```python
from build123d import *

# Parameters (mm, degrees)
SKETCH1_R           = 75
SKETCH1_R_2         = 4.5
BOSS_EXTRUDE1_DEPTH = 10
SKETCH2_R           = 30
BOSS_EXTRUDE2_DEPTH = 55
SKETCH3_R           = 40
BOSS_EXTRUDE3_DEPTH = 5
SKETCH4_R           = 22.5
CUT_EXTRUDE1_DEPTH  = 60
FILLET1_R           = 5
SKETCH5_W           = 40
SKETCH5_H           = 75
BOSS_EXTRUDE4_DEPTH = 45
CUT_EXTRUDE2_DEPTH  = 113.5
SKETCH7_R           = 30
BOSS_EXTRUDE5_DEPTH = 15
FILLET2_R           = 5
CUT_EXTRUDE3_DEPTH  = 45


with BuildPart() as part:
    # Sketch1 → Boss-Extrude1 (new body)
    with BuildSketch(Plane(origin=(0, 0, 0), x_dir=(1, 0, 0), z_dir=(0, 1, 0))):
        Circle(SKETCH1_R)
        with Locations((37.5, 37.5)):
            Circle(SKETCH1_R_2, mode=Mode.SUBTRACT)
        with Locations((-37.5, 37.5)):
            Circle(SKETCH1_R_2, mode=Mode.SUBTRACT)
        with Locations((-37.5, -37.5)):
            Circle(SKETCH1_R_2, mode=Mode.SUBTRACT)
        with Locations((37.5, -37.5)):
            Circle(SKETCH1_R_2, mode=Mode.SUBTRACT)
    extrude(amount=BOSS_EXTRUDE1_DEPTH)

    # Sketch2 → Boss-Extrude2 (add)
    with BuildSketch(Plane(origin=(0, 10, 0), x_dir=(1, 0, 0), z_dir=(0, 1, 0))):
        Circle(SKETCH2_R)
    extrude(amount=BOSS_EXTRUDE2_DEPTH)

    # Sketch3 → Boss-Extrude3 (add)
    with BuildSketch(Plane(origin=(0, 65, 0), x_dir=(1, 0, 0), z_dir=(0, 1, 0))):
        Circle(SKETCH3_R)
    extrude(amount=BOSS_EXTRUDE3_DEPTH)

    # Sketch4 → Cut-Extrude1 (cut)
    with BuildSketch(Plane(origin=(0, 70, 0), x_dir=(1, 0, 0), z_dir=(0, 1, 0))):
        Circle(SKETCH4_R)
    extrude(amount=-CUT_EXTRUDE1_DEPTH, mode=Mode.SUBTRACT)

    # Fillet1
    fillet1_edges = [part.edges().sort_by_distance(p)[0] for p in [
        (-30, 10, 0),
        (-30, 65, 0),
    ]]
    fillet(fillet1_edges, radius=FILLET1_R)

    # Sketch5 → Boss-Extrude4 (add)
    with BuildSketch(Plane(origin=(0, 10, 0), x_dir=(1, 0, 0), z_dir=(0, 1, 0))):
        with Locations((37.5, 0)):
            Rectangle(SKETCH5_W, SKETCH5_H)
    extrude(amount=BOSS_EXTRUDE4_DEPTH)

    # Sketch6 → Cut-Extrude2 (cut, through all)
    with BuildSketch(Plane.XY.offset(37.5)):
        Polygon((57.5, 25), (30, 25), (17.5, 25), (17.5, 10), (33, 10), (42, 10), (57.5, 10), align=None)
    extrude(amount=-CUT_EXTRUDE2_DEPTH, mode=Mode.SUBTRACT)

    # Sketch7 → Boss-Extrude5 (add)
    with BuildSketch(Plane(origin=(0, 10, 0), x_dir=(1, 0, 0), z_dir=(0, 1, 0))):
        Circle(SKETCH7_R)
    extrude(amount=BOSS_EXTRUDE5_DEPTH)

    # Fillet2
    fillet2_edges = [part.edges().sort_by_distance(p)[0] for p in [
        (26.69269563, 10, 13.693063938),
    ]]
    fillet(fillet2_edges, radius=FILLET2_R)

    # Sketch8 → Cut-Extrude3 (cut)
    with BuildSketch(Plane(origin=(0, 70, 0), x_dir=(1, 0, 0), z_dir=(0, 1, 0))):
        with BuildLine():
            ThreePointArc((17.5, 14.142135624), (-22.5, 0), (17.5, -14.142135624))
            ThreePointArc((17.5, -14.142135624), (22.5, 0), (17.5, 14.142135624))
        make_face()
    extrude(amount=-CUT_EXTRUDE3_DEPTH, mode=Mode.SUBTRACT)


solid = part.part
```
Input: part model. Units: mm. Frame: model coordinates. A direction names the side the tool comes from. Give positions to 0.01 mm unless a question says otherwise; leave off trailing zeros. Order: outer loops, then holes, each group sorted by start corner. A loop starts at its lowest first (then second) coordinate and runs counter-clockwise, first axis right, second up.
1. Cut plane A-A (y = 38.5). Return loops of the section in (x, z).
Computed:
outline: (17.5, -37.5) - (57.5, -37.5) - (57.5, 37.5) - (17.5, 37.5) - (17.5, 24.37) arc R30 ccw (long way) to (17.5, -24.37) - close; hole circle Ø45 at (0, 0)
2. Cut plane B-B (x = -37.5). Return loops of the section in (y, z), and give its area (3 significant figures).
Computed:
outline: (0, -64.95) - (10, -64.95) - (10, -42) - (0, -42) - close; (0, -33) - (10, -33) - (10, 33) - (0, 33) - close; (0, 42) - (10, 42) - (10, 64.95) - (0, 64.95) - close; (65, -13.92) - (70, -13.92) - (70, 13.92) - (65, 13.92) - close
area: 1,260 mm2
3. Line query: probe 1 along Z at (x, y) = (-37, 4); probe 2 along Y at (x, z) = (-26, 25.5); probe 3 along X at (y, z) = (59, 0). Output: solid intervals per line, ascending.
Computed:
probe 1: z = -65.24 to -41.97, -33.03 to 33.03, 41.97 to 65.24
probe 2: y = 0 to 10, 65 to 70
probe 3: x = -30 to -22.5, 22.5 to 30
4. Pin query (flat end, axial travel): pin 1 Ø1.5 at (x, y) = (5.5, 47) entering from +Z; pin 2 Ø10.5 at (y, z) = (46.5, 30.5) entering from -X; pin 3 Ø1 at (y, z) = (48.5, -34) entering from +X. Return the tip coordinate at first contact, or that it passes through.
Computed:
pin 1: stops at z = 29.62
pin 2: stops at x = -16.2
pin 3: stops at x = 57.5
5. Draft query along Y for faces 5 (the face through (42, 25, 1)), 6 (the face through (17.5, 13, -27)), 7 (the face through (-9.764, 4.93, -74.362)), 8 (the face through (0, 25, 0)). Return one class per face: released by +Y, released by -Y, zero draft, split by the parting line, or undercut.
Computed:
face 5: undercut
face 6: undercut
face 7: zero draft
face 8: released by +Y
6. Set-up query: faces 1 (the face through (57.5, 40, 1)), 2 (the face through (-0.2, 65, 35.4)), 3 (the face through (21.2, 47.82, 7.54)), 4 (the face through (37, 40, 37.5)). Return all of +Z, -Z, +X, -X, +Y, -Y with unobstructed straight access to the full face (end or side cutting, diameter ignored); none if empty.
Computed:
face 1: +Z, -Z, +X, +Y
face 2: none
face 3: +Y
face 4: +Z, +X, -X, +Y
7. Cut plane C-C (x = 51). Return loops of the section in (y, z), and give its area (3 significant figures).
Computed:
outline: (0, -54.99) - (10, -54.99) - (10, 54.99) - (0, 54.99) - close; (25, -37.5) - (55, -37.5) - (55, 37.5) - (25, 37.5) - close
area: 3,350 mm2
8. Cut plane D-D (y = 7.5). Return loops of the section in (x, z), and give its area (3 significant figures).
Computed:
outline: circle Ø150 at (0, 0); hole circle Ø9 at (-37.5, -37.5); hole circle Ø9 at (-37.5, 37.5); hole circle Ø9 at (37.5, -37.5); hole circle Ø9 at (37.5, 37.5)
area: 17,400 mm2
